For this review, take the finished solid that the model builds, in its own axes (mm). A direction names the side the tool comes from. Round coordinates to 2 decimals unless told otherwise and drop trailing zeros. Order: outer loops, then holes, each group sorted by start corner. A loop starts at its lowest first (then second) coordinate and runs counter-clockwise, first axis right, second up. Notation, with made-up numbers: M 82.25,-16 L 120.25,-16 A28 ccw 120.25,23 Z; hole C 60.5,29.25 d1. An arc over 180 degrees is marked long. Answer in a Markdown table with one row per item. Add a question column.
```python
from build123d import *

# Parameters (mm, degrees)
SKETCH1_R           = 45
BOSS_EXTRUDE1_DEPTH = 40
SKETCH2_R           = 39.5
BOSS_EXTRUDE2_DEPTH = 45
SKETCH3_R           = 5
BOSS_EXTRUDE3_DEPTH = 6.8
FILLET1_R           = 5


with BuildPart() as part:
    # Sketch1 → Boss-Extrude1 (new body)
    with BuildSketch(Plane(origin=(0, 0, 0), x_dir=(1, 0, 0), z_dir=(0, 1, 0))):
        Circle(SKETCH1_R)
    extrude(amount=BOSS_EXTRUDE1_DEPTH)

    # Sketch2 → Boss-Extrude2 (add)
    with BuildSketch(Plane(origin=(0, 40, 0), x_dir=(1, 0, 0), z_dir=(0, 1, 0))):
        Circle(SKETCH2_R)
    extrude(amount=BOSS_EXTRUDE2_DEPTH)

    # Sketch3 → Boss-Extrude3 (add)
    with BuildSketch(Plane(origin=(0, 85, 0), x_dir=(1, 0, 0), z_dir=(0, 1, 0))):
        Circle(SKETCH3_R)
    extrude(amount=BOSS_EXTRUDE3_DEPTH)

    # Fillet1
    fillet1_edges = [part.edges().sort_by_distance(p)[0] for p in [
        (-45, 0, 0),
        (-45, 40, 0),
        (-39.5, 85, 0),
    ]]
    fillet(fillet1_edges, radius=FILLET1_R)


solid = part.part
```
1. Consider section B-B on x = 0. Write out the cut boundary in (y, z).
2. Consider section D-D on y = 30. Write out the cut boundary in (x, z).
3. For faces 1 (the cylindrical face through (-1.08, 88.35, 4.88)), 2 (the flat face through (0, 91.8, 0)), list the 3-axis set-ups (+Z, -Z, +X, -X, +Y, -Y) from which the entire face can be reached by the end or side of a thin tool; tool diameter is ignored.
4. Clearance check with flat-ended pins moving along their axes: pin 1 Ø10 at (y, z) = (40.5, 0.5) entering from -X; pin 2 Ø2 at (x, y) = (10, 78) entering from -Z; pin 3 Ø6 at (x, y) = (30.5, 11) entering from +Z. State where each tip first meets the part, or that it passes through.
5. To check wall thickness, follow probe 1 along Y at (x, z) = (25.5, -6.5); probe 2 along Y at (x, z) = (27, 29); probe 3 along Z at (x, y) = (-10, 32.5). State the ranges of each line that lie inside material, in increasing order. Write a range as [from, to].
6. Consider section A-A on z = 0. Write out the cut boundary in (x, y), plus the area to 3 significant figures.
7. Consider section C-C on y = 71.5. Write out the cut boundary in (x, z).
Solved:
| question | item | result |
|---|---|---|
| 1 | outline | M 0,-40 A5 ccw 5,-45 L 35,-45 A5 ccw 40,-40 L 40,-39.5 L 80,-39.5 A5 ccw 85,-34.5 L 85,-5 L 91.8,-5 L 91.8,5 L 85,5 L 85,34.5 A5 ccw 80,39.5 L 40,39.5 L 40,40 A5 ccw 35,45 L 5,45 A5 ccw 0,40 Z |
| 2 | outline | C 0,0 d90 |
| 3 | face 1 | +Y |
| 3 | face 2 | +Z, -Z, +X, -X, +Y |
| 4 | pin 1 | stops at x = -44.97 |
| 4 | pin 2 | stops at z = -38.46 |
| 4 | pin 3 | stops at z = 35.62 |
| 5 | probe 1 | y = [0, 85] |
| 5 | probe 2 | y = [0, 40] |
| 5 | probe 3 | z = [-43.87, 43.87] |
| 6 | outline | M -45,5 A5 ccw -40,0 L 40,0 A5 ccw 45,5 L 45,35 A5 ccw 40,40 L 39.5,40 L 39.5,80 A5 ccw 34.5,85 L 5,85 L 5,91.8 L -5,91.8 L -5,85 L -34.5,85 A5 ccw -39.5,80 L -39.5,40 L -40,40 A5 ccw -45,35 Z |
| 6 | area | 7,190 mm^2 |
| 7 | outline | C 0,0 d79 |
